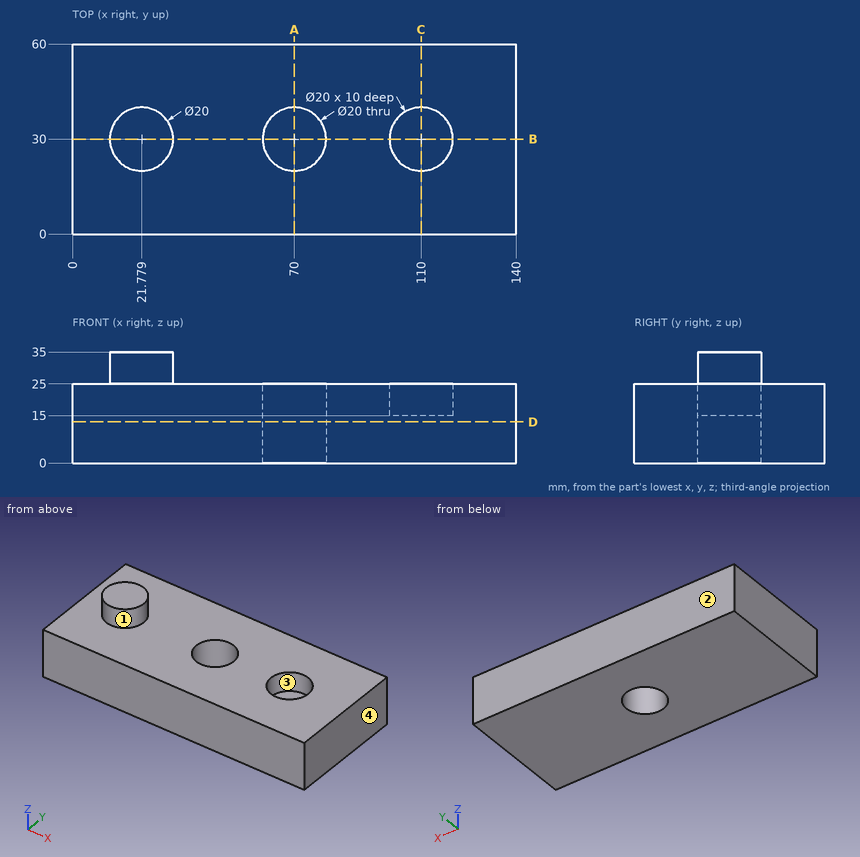
Source: three-view drawing plus pictorial views. Frame: mm from the lowest corner of the part. Give positions to 0.01 mm unless a question says otherwise; leave off trailing zeros. Loops run counter-clockwise (first coordinate to the right, second up) from the corner with the lowest first, then second, coordinate; pieces in that order, holes last. Notation, with made-up numbers: (78, -34.75) -> (87, -34.75) arc R14 cw to (87, -15.75) -> close; hole circle Ø6 at (57.5, 61). An arc over 180 degrees is marked (long way). Put each result on its own line as item: value. Start each with the question number.
1) Draft query along Y for the marked faces 1, 2, 3 and 4. Return one class per face: released by +Y, released by -Y, zero draft, split by the parting line, or undercut.
2) Cut plane B-B (y = 30). Return loops of the section in (x, z), then the cut area to 3 significant figures.
3) Cut plane D-D (z = 13). Return loops of the section in (x, y), then the cut area to 3 significant figures.
4) Material intervals for probe 1 along Y at (x, z) = (70, 8.5); probe 2 along X at (y, z) = (35.5, 18); probe 3 along Z at (x, y) = (122.5, 19.5), sorted ascending.
5) Cut plane A-A (x = 70). Return loops of the section in (y, z), then the cut area to 3 significant figures.
6) Cut plane C-C (x = 110). Return loops of the section in (y, z).
7) Contact query for flat-ended pins moving along their axis: P1, Ø23, axis at x = 70, y = 30, coming from the +Z side; P2, Ø1, axis at y = 28, z = 26, coming from the -X side; P3, Ø10, axis at x = 107, y = 27, coming from the +Z side. Output: stop coordinate, or through.
Results are:
1. face 1: split by the parting line
1. face 2: released by +Y
1. face 3: undercut
1. face 4: zero draft
2. outline: (0, 0) -> (60, 0) -> (60, 25) -> (31.78, 25) -> (31.78, 35) -> (11.78, 35) -> (11.78, 25) -> (0, 25) -> close; (80, 0) -> (140, 0) -> (140, 25) -> (120, 25) -> (120, 15) -> (100, 15) -> (100, 25) -> (80, 25) -> close
2. area: 3,000 mm2
3. outline: (0, 0) -> (140, 0) -> (140, 60) -> (0, 60) -> close; hole circle Ø20 at (70, 30)
3. area: 8,090 mm2
4. probe 1: y = 0 to 20, 40 to 60
4. probe 2: x = 0 to 61.65, 78.35 to 101.65, 118.35 to 140
4. probe 3: z = 0 to 25
5. outline: (0, 0) -> (20, 0) -> (20, 25) -> (0, 25) -> close; (40, 0) -> (60, 0) -> (60, 25) -> (40, 25) -> close
5. area: 1,000 mm2
6. outline: (0, 0) -> (60, 0) -> (60, 25) -> (40, 25) -> (40, 15) -> (20, 15) -> (20, 25) -> (0, 25) -> close
7. P1: stops at z = 25
7. P2: stops at x = 11.89
7. P3: stops at z = 15
